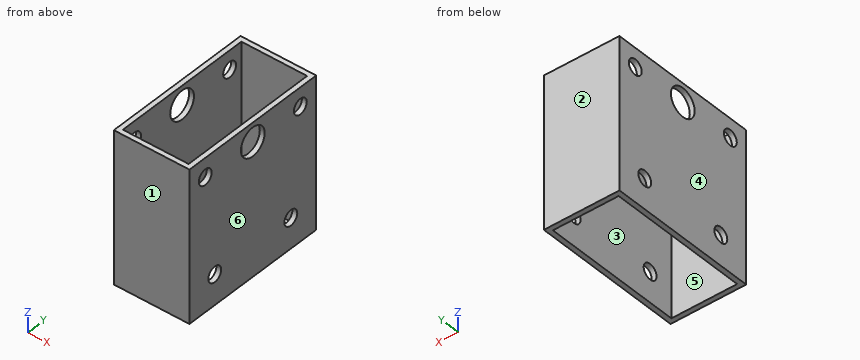
Autodesk Inventor part; units mm, degrees
ref_plane "YZ Plane" through (0, 0, 0) normal (1, 0, 0) x (0, 1, 0)
ref_plane "XZ Plane" through (0, 0, 0) normal (0, 1, 0) x (-1, 0, 0)
ref_plane "XY Plane" through (0, 0, 0) normal (0, 0, 1) x (1, 0, 0)
sketch "Sketch1" plane through (0, 0, 0) normal (0, 0, 1) x (1, 0, 0)
  line L0 (12.7, -25.4) -> (-12.7, -25.4)
  line L1 (-12.7, -25.4) -> (-12.7, 25.4)
  line L2 (-12.7, 25.4) -> (12.7, 25.4)
  line L3 (12.7, 25.4) -> (12.7, -25.4)
  line L4 (11.049, -23.749) -> (-11.049, -23.749)
  line L5 (-11.049, -23.749) -> (-11.049, 23.749)
  line L6 (-11.049, 23.749) -> (11.049, 23.749)
  line L7 (11.049, 23.749) -> (11.049, -23.749)
  dimension "d0" = 25.4
  dimension "d1" = 50.8
  dimension "d2" = 1.651
  dimension "d3" = 1.651
  dimension "d4" = 1.651
  dimension "d5" = 1.651
extrude "Extrusion1" add sketch "Sketch1" along normal blind 50.8
sketch "Sketch2" plane through (12.7, -25.4, 0) normal (1, 0, 0) x (0, 0, -1)
  circle A0 centre (-44.45, 25.4) radius 4.7625
  line L0 (-50.8, 0) -> (-50.8, 50.8)
  line L1 (0, 0) -> (-50.8, 0)
  point P0 (0, 25.4)
  dimension "d8" = 9.525
  dimension "d9" = 6.35
  dimension "d10" = 25.4
extrude "Extrusion2" cut sketch "Sketch2" against normal blind 50.8
sketch "Sketch3" plane through (12.7, -25.4, 0) normal (1, 0, 0) x (0, 0, -1)
  circle A0 centre (-10.16, 10.16) radius 2.5797
  circle A1 centre (-44.45, 6.35) radius 2.5797
  circle A2 centre (-44.45, 44.45) radius 2.5797
  circle A3 centre (-10.16, 40.64) radius 2.5797
  line L0 (0, 50.8) -> (-50.8, 50.8)
  line L1 (0, 50.8) -> (0, 0)
  line L2 (0, 0) -> (-50.8, 0)
  line L3 (-50.8, 0) -> (-50.8, 50.8)
  point P0 (0, 25.4)
  dimension "d13" = 10.16
  dimension "d14" = 10.16
  dimension "d15" = 6.35
  dimension "d16" = 6.35
  dimension "d17" = 6.35
  dimension "d18" = 6.35
  dimension "d19" = 10.16
  dimension "d20" = 10.16
  dimension "d21" = 5.1594
  dimension "d22" = 5.1594
  dimension "d23" = 5.1594
  dimension "d24" = 5.1594
extrude "Extrusion3" cut sketch "Sketch3" against normal blind 50.8 contours A0 | A1 | A2 | A3
equation "\"d3\" = d2"
equation "\"d5\" = d3"
equation "\"d14\" = d13"
equation "\"d16\" = d15"
equation "\"d17\" = d15"
equation "\"d18\" = d15"
equation "\"d19\" = d13"
equation "\"d20\" = d13"
equation "\"d22\" = d21"
equation "\"d23\" = d21"
equation "\"d24\" = d21"
properties part number "back support bearing holder"
Source: CAD feature listing. Evaluate the final solid. Frame: model axes, mm. Face numbers are marked on the shaded views. A direction names the side the tool comes from. Give positions to 0.01 mm unless a question says otherwise; leave off trailing zeros. Loops run counter-clockwise (first coordinate to the right, second up) from the corner with the lowest first, then second, coordinate; pieces in that order, holes last. Notation, with made-up numbers: (3.25, 46) -> (33.25, 46) arc R35 ccw to (33.25, 79) -> close; hole circle Ø1 at (-28.75, 38.5). An arc over 180 degrees is marked (long way). Put each result on its own line as item: value. Start each with the question number.
1) Reachability of the marked faces 5 and 6 from +Z, -Z, +X, -X, +Y, -Y: full face, straight path, thin tool, end or side. Return the list, or none.
2) Cut plane D-D (z = 44.45). State how many separate pieces and enclosed holes the cut face has, then the cut area to 3 significant figures.
3) Cut plane C-C (y = 19.05). Return loops of the section in (x, z).
4) Draft query along Y for the marked faces 1, 2, 3 and 4. Return one class per face: released by +Y, released by -Y, zero draft, split by the parting line, or undercut.
5) Material intervals for probe 1 along Y at (x, z) = (-12.4, 10.16); probe 2 along X at (y, z) = (-3.5, 3.5); probe 3 along Y at (x, z) = (-10.75, 21.5), sorted ascending.
6) Cut plane B-B (z = 10.16). Return loops of the section in (x, y), then the cut area to 3 significant figures.
7) Cut plane A-A (x = 4.25). Return loops of the section in (y, z).
Results are:
1. face 5: +Z, -Z
1. face 6: +Z, -Z, +X, +Y, -Y
2. separate pieces: 6
2. enclosed holes: 0
2. area: 175 mm2
3. outline: (-12.7, 0) -> (-11.05, 0) -> (-11.05, 41.87) -> (-12.7, 41.87) -> close; (-12.7, 47.03) -> (-11.05, 47.03) -> (-11.05, 50.8) -> (-12.7, 50.8) -> close; (11.05, 0) -> (12.7, 0) -> (12.7, 41.87) -> (11.05, 41.87) -> close; (11.05, 47.03) -> (12.7, 47.03) -> (12.7, 50.8) -> (11.05, 50.8) -> close
4. face 1: released by -Y
4. face 2: released by +Y
4. face 3: undercut
4. face 4: zero draft
5. probe 1: y = -25.4 to -17.82, -12.66 to 12.66, 17.82 to 25.4
5. probe 2: x = -12.7 to -11.05, 11.05 to 12.7
5. probe 3: y = -25.4 to -23.75, 23.75 to 25.4
6. outline: (-12.7, -25.4) -> (12.7, -25.4) -> (12.7, -17.82) -> (11.05, -17.82) -> (11.05, -23.75) -> (-11.05, -23.75) -> (-11.05, -17.82) -> (-12.7, -17.82) -> close; (-12.7, -12.66) -> (-11.05, -12.66) -> (-11.05, 12.66) -> (-12.7, 12.66) -> close; (-12.7, 17.82) -> (-11.05, 17.82) -> (-11.05, 23.75) -> (11.05, 23.75) -> (11.05, 17.82) -> (12.7, 17.82) -> (12.7, 25.4) -> (-12.7, 25.4) -> close; (11.05, -12.66) -> (12.7, -12.66) -> (12.7, 12.66) -> (11.05, 12.66) -> close
6. area: 207 mm2
7. outline: (-25.4, 0) -> (-23.75, 0) -> (-23.75, 50.8) -> (-25.4, 50.8) -> close; (23.75, 0) -> (25.4, 0) -> (25.4, 50.8) -> (23.75, 50.8) -> close
